Part model, mm, in its own coordinate system. A direction names the side the tool comes from. Coordinates: 2 decimals unless noted, no trailing zeros. Write each loop counter-clockwise with the first axis right and the second up, starting at its lowest first coordinate (ties: lowest second). Pieces come first, ordered by that corner, then holes. Notation, with made-up numbers: (-32, -8.5) - (6, -8.5) arc R20 ccw to (6, 19.5) - close; hole circle Ø5 at (5, -4.5). An arc over 180 degrees is marked (long way). Use one line per item in the form item = value. Start each with the question number.
from build123d import *

# Parameters (mm, degrees)
SKETCH1_W            = 6.266
SKETCH1_H            = 19.6
SKETCH1_R            = 1.675
SKETCH1_W_2          = 52.832
SKETCH1_H_2          = 5
BOSS_EXTRUDE2_DEPTH  = 3.175
SKETCH3_W            = 30
SKETCH3_H            = 29.6
BOSS_EXTRUDE3_DEPTH  = 3.175
SKETCH4_R            = 4.75
CUT_EXTRUDE1_DEPTH   = 10
BOSS_EXTRUDE14_DEPTH = 3.175
CUT_EXTRUDE8_DEPTH   = 10
BOSS_EXTRUDE15_DEPTH = 3.175
BOSS_EXTRUDE16_DEPTH = 3.175
BOSS_EXTRUDE17_DEPTH = 3.175
FILLET5_R            = 4
SKETCH27_W           = 3.175
SKETCH27_H           = 8
CUT_EXTRUDE9_DEPTH   = 10
SKETCH28_W           = 18
SKETCH28_H           = 3.175
BOSS_EXTRUDE18_DEPTH = 3.175
SKETCH29_W           = 53.813797415
SKETCH29_H           = 23.475817665
BOSS_EXTRUDE19_DEPTH = 3.175
SKETCH30_W           = 8.216536182
SKETCH30_H           = 11.169409555
BOSS_EXTRUDE20_DEPTH = 3.175


with BuildPart() as part:
    # Sketch1 → Boss-Extrude2 (new body)
    # profile 1 of 4: a face of its own
    with BuildSketch(Plane.XY):
        with Locations((-23.283, 0)):
            Rectangle(SKETCH1_W, SKETCH1_H)
        with Locations((-23.95, -4.974)):
            Circle(SKETCH1_R, mode=Mode.SUBTRACT)
        with Locations((-23.95, 4.974)):
            Circle(SKETCH1_R, mode=Mode.SUBTRACT)
    # profile 2 of 4: a face of its own
    with BuildSketch(Plane.XY):
        with Locations((23.283, 0)):
            Rectangle(SKETCH1_W, SKETCH1_H)
        with Locations((23.95, -4.974)):
            Circle(SKETCH1_R, mode=Mode.SUBTRACT)
        with Locations((23.95, 4.974)):
            Circle(SKETCH1_R, mode=Mode.SUBTRACT)
    # profile 3 of 4: a face of its own
    with BuildSketch(Plane.XY):
        with Locations((0, 12.3)):
            Rectangle(SKETCH1_W_2, SKETCH1_H_2)
    # profile 4 of 4: a face of its own
    with BuildSketch(Plane.XY):
        with Locations((0, -12.3)):
            Rectangle(SKETCH1_W_2, SKETCH1_H_2)
    extrude(amount=BOSS_EXTRUDE2_DEPTH)

    # Sketch3 → Boss-Extrude3 (add)
    with BuildSketch(Plane.XY.offset(3.175)):
        with Locations((41.416, 0)):
            Rectangle(SKETCH3_W, SKETCH3_H)
    extrude(amount=-BOSS_EXTRUDE3_DEPTH)

    # Sketch4 → Cut-Extrude1 (cut)
    with BuildSketch(Plane(origin=(0, 0, 0), x_dir=(-1, 0, 0), z_dir=(0, 0, -1))):
        with Locations((-40.576, 7.77)):
            Circle(SKETCH4_R)
    extrude(amount=-CUT_EXTRUDE1_DEPTH, mode=Mode.SUBTRACT)

    # Sketch22 → Boss-Extrude14 (add)
    with BuildSketch(Plane(origin=(0, 0, 0), x_dir=(-1, 0, 0), z_dir=(0, 0, -1))):
        with BuildLine():
            ThreePointArc((-34.680262133, 14.8), (-40.576, 16.945), (-46.471737867, 14.8))
            Line((-46.471737867, 14.8), (-34.680262133, 14.8))
        make_face()
    extrude(amount=-BOSS_EXTRUDE14_DEPTH)

    # Sketch23 → Cut-Extrude8 (cut)
    with BuildSketch(Plane(origin=(0, 0, 0), x_dir=(-1, 0, 0), z_dir=(0, 0, -1))):
        with BuildLine():
            Line((-49.751, -14.8), (-49.751, 7.77))
            ThreePointArc((-49.751, 7.77), (-48.890866804, 11.648609936), (-46.471737867, 14.8))
            Line((-46.471737867, 14.8), (-56.416, 14.8))
            Line((-56.416, 14.8), (-56.416, -14.8))
            Line((-56.416, -14.8), (-49.751, -14.8))
        make_face()
    extrude(amount=-CUT_EXTRUDE8_DEPTH, mode=Mode.SUBTRACT)

    # Sketch24 → Boss-Extrude15 (add)
    with BuildSketch(Plane(origin=(0, 0, 0), x_dir=(-1, 0, 0), z_dir=(0, 0, -1))):
        Polygon((30.625, 14.8), (26.416, 14.8), (26.416, -14.8), (27.751006616, -14.8), (30.625, -14.8), align=None)
    extrude(amount=-BOSS_EXTRUDE15_DEPTH)

    # Sketch25 → Boss-Extrude16 (add)
    with BuildSketch(Plane(origin=(0, 0, 0), x_dir=(-1, 0, 0), z_dir=(0, 0, -1))):
        Polygon((30.625, 14.8), (30.625, 9.8), (33.8, 9.8), (33.8, 1.8), (30.625, 1.8), (30.625, -1.8), (33.8, -1.8), (33.8, -9.8), (30.625, -9.8), (30.625, -14.8), (31.879074074, -14.8), (38.8, -14.8), (38.8, 14.8), align=None)
    extrude(amount=-BOSS_EXTRUDE16_DEPTH)

    # Sketch26 → Boss-Extrude17 (add)
    with BuildSketch(Plane(origin=(0, 0, 0), x_dir=(-1, 0, 0), z_dir=(0, 0, -1))):
        with BuildLine():
            ThreePointArc((-40.225848077, 16.938316019), (-37.275108655, 16.330650754), (-34.680262133, 14.8))
            Line((-34.680262133, 14.8), (38.8, 14.8))
            ThreePointArc((38.8, 14.8), (-0.708684686, 16.025831975), (-40.225848077, 16.938316019))
        make_face()
    extrude(amount=-BOSS_EXTRUDE17_DEPTH)

    # Fillet5
    fillet5_edges = [part.edges().sort_by_distance(p)[0] for p in [
        (-38.8, 14.8, 1.5875),
    ]]
    fillet(fillet5_edges, radius=FILLET5_R)

    # Sketch27 → Cut-Extrude9 (cut)
    with BuildSketch(Plane(origin=(0, 0, 0), x_dir=(-1, 0, 0), z_dir=(0, 0, -1))):
        with Locations((-43.1635, -5.8)):
            Rectangle(SKETCH27_W, SKETCH27_H)
    extrude(amount=-CUT_EXTRUDE9_DEPTH, mode=Mode.SUBTRACT)

    # Sketch28 → Boss-Extrude18 (add)
    with BuildSketch(Plane(origin=(0, 0, 0), x_dir=(-1, 0, 0), z_dir=(0, 0, -1))):
        with Locations((-40.751, -16.3875)):
            Rectangle(SKETCH28_W, SKETCH28_H)
        with Locations((-5.45, -16.3875)):
            Rectangle(SKETCH28_W, SKETCH28_H)
        with Locations((29.8, -16.3875)):
            Rectangle(SKETCH28_W, SKETCH28_H)
    extrude(amount=-BOSS_EXTRUDE18_DEPTH)

    # Sketch29 → Boss-Extrude19 (add)
    with BuildSketch(Plane(origin=(0, 0, 0), x_dir=(-1, 0, 0), z_dir=(0, 0, -1))):
        with Locations((0.393454416, 0.74908249)):
            Rectangle(SKETCH29_W, SKETCH29_H)
    extrude(amount=-BOSS_EXTRUDE19_DEPTH)

    # Sketch30 → Boss-Extrude20 (add)
    with BuildSketch(Plane(origin=(0, 0, 0), x_dir=(-1, 0, 0), z_dir=(0, 0, -1))):
        with Locations((-41.72757997, -5.584704778)):
            Rectangle(SKETCH30_W, SKETCH30_H)
    extrude(amount=-BOSS_EXTRUDE20_DEPTH)


solid = part.part
Q1. Which spindle directions (+Z, -Z, +X, -X, +Y, -Y) get a long thin tool onto all of the face, cutting with end or side? Do faces 4 (the flat face through (-30, -17.975, 2)), 5 (the flat face through (-32, -1.8, 2)), 6 (the cylindrical face through (2.115, 16.064, 1.565)), 7 (the flat face through (-3.55, -16, 2)). Say none if no direction does.
Q2. Drill centre lines: probe 1 along X at (y, z) = (-16, 2.05); probe 2 along X at (y, z) = (4, 0.4) (3 decimals); probe 3 along X at (y, z) = (2, 3.05) (3 decimals). Where is each one in solid material? Low to high.
Q3. Pin check, flat tips, straight feed: P1, Ø1, axis at x = 24.5, z = 1.5, coming from the -Y side; P2, Ø1.5, axis at x = 15.5, z = 0.5, coming from the +Y side; P3, Ø1.6, axis at x = -32, z = 1, coming from the +Y side. Stop position of each tip, or through.
Q4. Slice it at A-A (z = 0.75). List the corners of the cut face in (x, y) (3 decimals).
Q5. Slice it at B-B (y = -7.5). List the corners of the cut face in (x, z) (3 decimals), plus the area to 3 significant figures.
Q6. Mould opens along Y. For faces 1 (the cylindrical face through (-37.646, 13.746, 1.61)), 2 (the flat face through (-32, -9.8, 2)), 3 (the flat face through (-20.8, -16, 2)) say: released by +Y, released by -Y, zero draft, split by the parting line, or undercut.
Q7. Slice it at C-C (x = 17). List the corners of the cut face in (y, z) (3 decimals), plus the area to 3 significant figures.
Q8. Slice it at D-D (y = 14). List the corners of the cut face in (x, z) (3 decimals).
Solution:
q1.face_4 = +Z, -Z, +X, -X, -Y
q1.face_5 = +Z, -Z
q1.face_6 = +Z, -Z, -X, +Y
q1.face_7 = +Z, -Z, -Y
q2.probe_1 = -38.8 to -20.8, -3.55 to 14.45, 31.75 to 49.75
q2.probe_2 = -38.8 to -33.8, -30.625 to 37.686, 43.466 to 49.751
q2.probe_3 = -38.8 to -33.8, -30.625 to 49.751
q3.P1 = -14.8
q3.P2 = 16.42
q3.P3 = 15.06
q4.outline = (-38.8, -17.975) - (-20.8, -17.975) - (-20.8, -14.8) - (-3.55, -14.8) - (-3.55, -17.975) - (14.45, -17.975) - (14.45, -14.8) - (31.751, -14.8) - (31.751, -17.975) - (49.751, -17.975) - (49.751, 7.77) arc R9.175 ccw to (40.226, 16.938) arc R4984.45 ccw to (-34.937, 14.934) arc R4 ccw to (-38.8, 10.936) - close; hole (-33.8, -9.8) - (-30.625, -9.8) - (-30.625, -1.8) - (-33.8, -1.8) - close; hole (-33.8, 1.8) - (-30.625, 1.8) - (-30.625, 9.8) - (-33.8, 9.8) - close; hole circle Ø9.5 at (40.576, 7.77)
q5.outline = (-38.8, 0) - (-33.8, 0) - (-33.8, 3.175) - (-38.8, 3.175) - close; (-30.625, 0) - (49.751, 0) - (49.751, 3.175) - (-30.625, 3.175) - close
q5.area = 271 mm2
q6.face_1 = released by +Y
q6.face_2 = undercut
q6.face_3 = zero draft
q7.outline = (-14.8, 0) - (16.44, 0) - (16.44, 3.175) - (-14.8, 3.175) - close
q7.area = 99.2 mm2
q8.outline = (-37.371, 0) - (47.312, 0) - (47.312, 3.175) - (-37.371, 3.175) - close
